Build history of the part. All positions in model axes, mm. A direction names the side the tool comes from. Give positions to 0.01 mm unless a question says otherwise; leave off trailing zeros. Order: outer loops, then holes, each group sorted by start corner. A loop starts at its lowest first (then second) coordinate and runs counter-clockwise, first axis right, second up. Notation, with made-up numbers: (49, 46.25) -> (100, 46.25) arc R27 cw to (100, 85.25) -> close; hole circle Ø7 at (-28.5, 81.5). An arc over 180 degrees is marked (long way). One line per question, with ' | ' between items. Start each with the question number.
(1) Cut at D-D (z = -20). Give the cut face in (x, y).
(2) Drill centre lines: L1, parallel to Z at x = 38, y = 4.5; L2, parallel to Z at x = 59, y = 9.5; L3, parallel to X at y = 5.25, z = -9.5. Where is each one in solid material? Low to high. Write a range as from..to.
(3) Which spindle directions (+Z, -Z, +X, -X, +Y, -Y) get a long thin tool onto all of the face, cutting with end or side? Do faces 1 (the face through (2, 9, -6.25)), 2 (the face through (1.232, 8.209, -14.248)), 3 (the face through (27.5, 0.5, -8.7)). Say none if no direction does.
(4) Cut at A-A (y = 6.25). Give the cut face in (x, z), then the cut area to 3 significant figures.
(5) Cut at C-C (x = 33). Give the cut face in (y, z).
(6) Cut at B-B (z = -31). Give the cut face in (x, y).
(7) Pull direction X, two halves, no side cores. Call faces 4 (the face through (1, 5, -2)), 5 (the face through (28, 10, -40)), 6 (the face through (47, 9, -1.25)): +X half, -X half, draft (parallel to the pull), parting line (faces both ways), or undercut.
(8) Pin check, flat tips, straight feed: pin 1 Ø1.1 at (x, y) = (2, 9) entering from -Z; pin 2 Ø5 at (x, z) = (57.5, -21) entering from +Y; pin 3 Ø0.8 at (y, z) = (9, -1.5) entering from -X; pin 4 Ø12 at (x, z) = (28, -32.5) entering from -Y. Stop position of each tip, or through.
from build123d import *

# Parameters (mm, degrees)
BOSS_EXTRUDE1_DEPTH      = 10
BOSS_EXTRUDE2_DEPTH      = 2.5
CUT_EXTRUDE2_START       = -2
CUT_EXTRUDE2_DEPTH       = 2
BOSS_EXTRUDE3_DEPTH      = 1.9
BOSS_EXTRUDE3_DEPTH_BACK = 1.9
CUT_EXTRUDE3_DEPTH       = 5
CUT_EXTRUDE3_DEPTH_BACK  = 5
CUT_EXTRUDE4_DEPTH       = 10


with BuildPart() as part:
    # Sketch1 → Boss-Extrude1 (new body)
    with BuildSketch(Plane(origin=(0, 0, 0), x_dir=(1, 0, 0), z_dir=(0, 1, 0))):
        with BuildLine():
            Line((5, 0), (60, 0))
            ThreePointArc((60, 0), (63.535533906, 1.464466094), (65, 5))
            Line((65, 5), (65, 36))
            ThreePointArc((65, 36), (63.535533906, 39.535533906), (60, 41))
            Line((60, 41), (5, 41))
            ThreePointArc((5, 41), (1.464466094, 39.535533906), (0, 36))
            Line((0, 36), (0, 5))
            ThreePointArc((0, 5), (1.464466094, 1.464466094), (5, 0))
        make_face()
        with BuildLine():
            Line((7.5, 38.5), (57.5, 38.5))
            ThreePointArc((57.5, 38.5), (61.035533906, 37.035533906), (62.5, 33.5))
            Line((62.5, 33.5), (62.5, 7.5))
            ThreePointArc((62.5, 7.5), (61.035533906, 3.964466094), (57.5, 2.5))
            Line((57.5, 2.5), (7.5, 2.5))
            ThreePointArc((7.5, 2.5), (3.964466094, 3.964466094), (2.5, 7.5))
            Line((2.5, 7.5), (2.5, 33.5))
            ThreePointArc((2.5, 33.5), (3.964466094, 37.035533906), (7.5, 38.5))
        make_face(mode=Mode.SUBTRACT)
    extrude(amount=BOSS_EXTRUDE1_DEPTH)

    # Sketch2 → Boss-Extrude2 (add)
    with BuildSketch(Plane(origin=(0, 0, 0), x_dir=(1, 0, 0), z_dir=(0, 1, 0))):
        with BuildLine():
            Line((7.5, 38.5), (57.5, 38.5))
            ThreePointArc((57.5, 38.5), (61.035533906, 37.035533906), (62.5, 33.5))
            Line((62.5, 33.5), (62.5, 7.5))
            ThreePointArc((62.5, 7.5), (61.035533906, 3.964466094), (57.5, 2.5))
            Line((57.5, 2.5), (7.5, 2.5))
            ThreePointArc((7.5, 2.5), (3.964466094, 3.964466094), (2.5, 7.5))
            Line((2.5, 7.5), (2.5, 33.5))
            ThreePointArc((2.5, 33.5), (3.964466094, 37.035533906), (7.5, 38.5))
        make_face()
    extrude(amount=BOSS_EXTRUDE2_DEPTH)

    # Sketch4 → Cut-Extrude2 (cut)
    with BuildSketch(Plane(origin=(0, 10, 0), x_dir=(1, 0, 0), z_dir=(0, 1, 0)).offset(CUT_EXTRUDE2_START)):
        with BuildLine():
            Line((6.25, 39.75), (58.75, 39.75))
            ThreePointArc((58.75, 39.75), (62.285533906, 38.285533906), (63.75, 34.75))
            Line((63.75, 34.75), (63.75, 6.25))
            ThreePointArc((63.75, 6.25), (62.285533906, 2.714466094), (58.75, 1.25))
            Line((58.75, 1.25), (6.25, 1.25))
            ThreePointArc((6.25, 1.25), (2.714466094, 2.714466094), (1.25, 6.25))
            Line((1.25, 6.25), (2.658770817, 6.25))
            ThreePointArc((2.658770817, 6.25), (4.438137822, 3.547152925), (7.5, 2.5))
            Line((7.5, 2.5), (57.5, 2.5))
            ThreePointArc((57.5, 2.5), (61.035533906, 3.964466094), (62.5, 7.5))
            Line((62.5, 7.5), (62.5, 33.5))
            ThreePointArc((62.5, 33.5), (61.035533906, 37.035533906), (57.5, 38.5))
            Line((57.5, 38.5), (7.5, 38.5))
            ThreePointArc((7.5, 38.5), (4.438137822, 37.452847075), (2.658770817, 34.75))
            Line((2.658770817, 34.75), (1.25, 34.75))
            ThreePointArc((1.25, 34.75), (2.714466094, 38.285533906), (6.25, 39.75))
        make_face()
    extrude(amount=CUT_EXTRUDE2_DEPTH, mode=Mode.SUBTRACT)

    # Sketch5 → Boss-Extrude3 (add, two sides: drawn at the far end of the back side and taken through both)
    with BuildSketch(Plane(origin=(32.5, 0, 0), x_dir=(0, 0, -1), z_dir=(1, 0, 0)).offset(-BOSS_EXTRUDE3_DEPTH_BACK)):
        with BuildLine():
            Line((1.25, 10), (1.25, 8))
            Line((1.25, 8), (1.81941821, 8.678606187))
            ThreePointArc((1.81941821, 8.678606187), (1.936395991, 8.999999993), (1.819418212, 9.3213938))
            Line((1.819418212, 9.3213938), (1.25, 10))
        make_face()
        with BuildLine():
            Line((39.180581788, 9.3213938), (39.75, 10))
            Line((39.75, 10), (39.75, 8))
            Line((39.75, 8), (39.18058179, 8.678606187))
            ThreePointArc((39.18058179, 8.678606187), (39.063604009, 8.999999993), (39.180581788, 9.3213938))
        make_face()
    extrude(amount=BOSS_EXTRUDE3_DEPTH + BOSS_EXTRUDE3_DEPTH_BACK)

    # Sketch6 → Cut-Extrude3 (cut, two sides: drawn at the far end of the back side and taken through both)
    with BuildSketch(Plane(origin=(32.5, 0, 0), x_dir=(0, 0, -1), z_dir=(1, 0, 0)).offset(-CUT_EXTRUDE3_DEPTH_BACK)):
        Polygon((10, 0), (8.75, 1.25), (7.5, 0), align=None)
    extrude(amount=CUT_EXTRUDE3_DEPTH + CUT_EXTRUDE3_DEPTH_BACK, mode=Mode.SUBTRACT)

    # Sketch3 → Cut-Extrude4 (cut)
    with BuildSketch(Plane(origin=(0, 0, 0), x_dir=(0, 0, -1), z_dir=(1, 0, 0))):
        with BuildLine():
            Line((25.000032513, 7.494104603), (15.999967487, 7.494104603))
            ThreePointArc((15.999967487, 7.494104603), (13.49407209, 10), (15.999967487, 12.505895397))
            Line((15.999967487, 12.505895397), (25.000032513, 12.505895397))
            ThreePointArc((25.000032513, 12.505895397), (27.50592791, 10), (25.000032513, 7.494104603))
        make_face()
    extrude(amount=CUT_EXTRUDE4_DEPTH, mode=Mode.SUBTRACT)


solid = part.part
Result set:
1) outline: (0, 0) -> (65, 0) -> (65, 10) -> (63.75, 10) -> (63.75, 8) -> (62.5, 8) -> (62.5, 2.5) -> (2.5, 2.5) -> (2.5, 7.49) -> (0, 7.49) -> close
2) L1: z = -41..-38.5, -2.5..0 | L2: z = -41..-39.74, -1.26..0 | L3: x = 0..2.5, 62.5..65
3) face 1: +Y | face 2: -X, +Y | face 3: -Y
4) outline: (0, -36) arc R5 ccw to (5, -41) -> (60, -41) arc R5 ccw to (65, -36) -> (65, -5) arc R5 ccw to (60, 0) -> (5, 0) arc R5 ccw to (0, -5) -> close; hole (2.5, -33.5) arc R5 ccw to (7.5, -38.5) -> (57.5, -38.5) arc R5 ccw to (62.5, -33.5) -> (62.5, -7.5) arc R5 ccw to (57.5, -2.5) -> (7.5, -2.5) arc R5 ccw to (2.5, -7.5) -> close | area: 505 mm2
5) outline: (0, -41) -> (10, -41) -> (10, -39.75) -> (9.32, -39.18) arc R0.5 ccw to (8.68, -39.18) -> (8, -39.75) -> (8, -38.5) -> (2.5, -38.5) -> (2.5, -2.5) -> (8, -2.5) -> (8, -1.25) -> (8.68, -1.82) arc R0.5 ccw to (9.32, -1.82) -> (10, -1.25) -> (10, 0) -> (0, 0) -> (0, -7.5) -> (1.25, -8.75) -> (0, -10) -> close
6) outline: (0, 0) -> (65, 0) -> (65, 10) -> (63.75, 10) -> (63.75, 8) -> (62.5, 8) -> (62.5, 2.5) -> (2.5, 2.5) -> (2.5, 10) -> (0, 10) -> close
7) face 4: -X half | face 5: draft | face 6: undercut
8) pin 1: stops at z = -40.36 | pin 2: stops at y = 2.5 | pin 3: stops at x = 1.08 | pin 4: stops at y = 0
